Could you check a few things on this model? Use its own coordinates, in mm. A direction names the side the tool comes from. Give positions to 0.01 mm unless a question says otherwise; leave off trailing zeros. Loops run counter-clockwise (first coordinate to the right, second up) from the corner with the lowest first, then second, coordinate; pieces in that order, holes last. Notation, with made-up numbers: M -16,60.5 L 14,60.5 A20 ccw 14,91.5 Z; hole C 15,-40 d10. An arc over 180 degrees is marked long. Answer in a Markdown table with one row per item. Add a question column.
1. Which directions (+Z, -Z, +X, -X, +Y, -Y) give clear straight access to the entire face, cutting with the end or side of a thin tool? Please do faces 4 (the flat face through (0, -9.994, -12)), 5 (the flat face through (-2, -6.494, 23)), 6 (the flat face through (24, -9, -3.544)).
2. I need wall thicknesses on line 1 along X through (y, z) = (-8.25, 17.5); line 2 along Z through (x, y) = (15.25, -7.05); line 3 along Z through (x, y) = (-18.5, -7.05). Which ranges of each line are inside material? Lowest first, please. Write a range as from..to.
3. If we section it at D-D on x = -19: List the corners of the cut face in (y, z) for me, then the cut area to 3 significant figures.
4. If we section it at B-B on z = 0: List the corners of the cut face in (x, y) for me (3 decimals).
5. If we section it at C-C on y = -9: List the corners of the cut face in (x, z) for me (3 decimals).
6. I'm going to push flat-ended pins straight in: pin 1 Ø2.5 at (x, y) = (-24.5, -10) entering from -Z; pin 2 Ø3.5 at (x, y) = (23.5, -9.5) entering from -Z; pin 3 Ø1.5 at (x, y) = (23.5, -10) entering from +Z. Where does each tip first touch, or does it pass through?
7. Thinking about a two-plate mould opening in X: for faces 1 (the flat face through (24, -10, 3.456)), 2 (the flat face through (10, -11.5, -19)), 3 (the cylindrical face through (-24.68, -13.34, -7.77)), which applies, released by +X, released by -X, zero draft, split by the parting line, or undercut?
8. If we section it at A-A on x = 0: List the corners of the cut face in (y, z) for me (3 decimals), then the cut area to 3 significant figures.
Autodesk Inventor part; units mm, degrees
ref_plane "Work Plane1" through (-28, 0, 0) normal (1, 0, 0) x (0, 1, 0)
ref_plane "Work Plane2" through (28, 0, 0) normal (1, 0, 0) x (0, 1, 0)
ref_plane "XZ Plane" through (0, 0, 0) normal (0, 1, 0) x (-1, 0, 0)
sketch "Sketch2" plane through (0, 0, 0) normal (0, 0, 1) x (1, 0, 0)
  line L0 (0, 0) -> (-20.875, 0)
  line L1 (-20.875, 0) -> (-20.875, -11.5)
  line L2 (-20.875, -11.5) -> (-22.875, -11.5)
  line L3 (-22.875, -11.5) -> (-22.875, -6.4943)
  line L4 (-22.875, -6.4943) -> (-25.875, -6.4943)
  line L5 (-25.875, -6.4943) -> (-25.875, -12.9943)
  line L6 (0, -3) -> (0, 0)
  line L7 (-25.875, -12.9943) -> (-25.875, -19.9943)
  line L8 (-25.875, -19.9943) -> (-14.1, -19.9943)
  line L9 (-14.1, 0) -> (-14.1, -19.9943) construction
  line L10 (-7.6, 0) -> (-7.6, -3) construction
  line L11 (-7.6, -3) -> (0, -3) construction
  line L12 (-7.6, 0) -> (-7.6, -10) construction
  line L13 (-8.349, -3) -> (-14.1, -3)
  line L14 (-14.1, -19.9943) -> (-14.1, -3)
  line L15 (-11.6, -3) -> (-11.6, -9.9943)
  line L16 (-11.6, -9.9943) -> (-14.1, -9.9943)
  line L17 (-7.6, 0) -> (-8.349, -3)
  dimension "d3" = 20.875
  dimension "d4" = 11.5
  dimension "d5" = 2
  dimension "d6" = 3
  dimension "d7" = 6.5
  dimension "d9" = 7
  dimension "d10" = 14.1
  dimension "d11" = 3
  dimension "d12" = 7.6
  dimension "d13" = 10
  dimension "d31" = 2.5
  dimension "d33" = 10
revolve "Revolution1" add sketch "Sketch2" angle 360 about axis through (0, -3, 0) along (0, 1, 0)
sketch "Sketch3" plane through (0, 0, 0) normal (1, 0, 0) x (0, 1, 0)
  line L0 (0, -7.6) -> (0, 7.6)
  circle A0 centre (-7.05, 0) radius 3.5
  point P0 (0, 0)
  dimension "d16" = 7.05
  dimension "d17" = 0
  dimension "d20" = 7
extrude "Extrusion1" cut sketch "Sketch3" along normal through all both and the other way through all
ref_plane "Work Plane1" through (-28, 0, 0) normal (1, 0, 0) x (0, 1, 0)
sketch "Sketch4" plane through (-28, 0, 0) normal (1, 0, 0) x (0, 1, 0)
  line L0 (-11.5, -20.875) -> (-11.5, 20.875)
  line L1 (-6.4943, -3.4556) -> (-11.5, -3.4556)
  line L2 (-11.5, -3.4556) -> (-11.5, 3.5444)
  line L3 (-11.5, 3.5444) -> (-6.4943, 3.5444)
  line L4 (-6.4943, 3.5444) -> (-6.4943, -3.4556)
  point P0 (0, 0)
  dimension "d24" = 7
extrude "Extrusion2" cut sketch "Sketch4" along normal up to surface
ref_plane "Work Plane2" through (28, 0, 0) normal (1, 0, 0) x (0, 1, 0)
sketch "Sketch5" plane through (28, 0, 0) normal (1, 0, 0) x (0, 1, 0)
  line L0 (-11.5, -20.875) -> (-11.5, 20.875)
  line L1 (-6.4943, 3.4556) -> (-11.5, 3.4556)
  line L2 (-11.5, 3.4556) -> (-11.5, -3.5444)
  line L3 (-11.5, -3.5444) -> (-6.4943, -3.5444)
  line L4 (-6.4943, -3.5444) -> (-6.4943, 3.4556)
  point P0 (0, 0)
  dimension "d28" = 7
extrude "Extrusion3" cut sketch "Sketch5" against normal up to surface
properties part number "bottom seal v2"
Results:
| question | item | result |
|---|---|---|
| 1 | face 4 | -Y |
| 1 | face 5 | +Z, +Y |
| 1 | face 6 | +X, +Y |
| 2 | line 1 | -19.06..-14.73, -11.38..11.38, 14.73..19.06 |
| 2 | line 2 | -20.9..-17.05, -14.25..-3.5, 3.5..14.25, 17.05..20.9 |
| 2 | line 3 | -18.09..-13.45, -9.67..-3.5, 3.5..9.67, 13.45..18.09 |
| 3 | outline | M -19.99,-17.56 L -6.49,-17.56 L -6.49,-12.74 L -11.5,-12.74 L -11.5,-8.65 L 0,-8.65 L 0,8.65 L -11.5,8.65 L -11.5,12.74 L -6.49,12.74 L -6.49,17.56 L -19.99,17.56 Z; hole C -7.05,0 d7 |
| 3 | area | 507 mm2 |
| 4 | outline | M -25.875,-19.994 L -14.1,-19.994 L -14.1,-10.55 L -20.875,-10.55 L -20.875,-11.5 L -25.875,-11.5 Z; M -20.875,-3.55 L -11.6,-3.55 L -11.6,-3 L -8.349,-3 L -7.6,0 L -20.875,0 Z; M 7.6,0 L 8.349,-3 L 11.6,-3 L 11.6,-3.55 L 20.875,-3.55 L 20.875,0 Z; M 14.1,-19.994 L 25.875,-19.994 L 25.875,-11.5 L 20.875,-11.5 L 20.875,-10.55 L 14.1,-10.55 Z |
| 5 | outline | M -25.643,-3.456 A25.875 ccw 25.631,-3.544 L 22.599,-3.544 A22.875 cw -22.612,-3.456 Z; M -25.631,3.544 L -22.599,3.544 A22.875 cw 22.612,3.456 L 25.643,3.456 A25.875 ccw Z; M -20.672,-2.906 A20.875 ccw 20.672,-2.906 L 11.23,-2.906 A11.6 cw -11.23,-2.906 Z; M -20.672,2.906 L -11.23,2.906 A11.6 cw 11.23,2.906 L 20.672,2.906 A20.875 ccw Z |
| 6 | pin 1 | z = -11.36 |
| 6 | pin 2 | z = -14.02 |
| 6 | pin 3 | z = 12.33 |
| 7 | face 1 | zero draft |
| 7 | face 2 | undercut |
| 7 | face 3 | split by the parting line |
| 8 | outline | M -19.994,-25.875 L -6.494,-25.875 L -6.494,-22.875 L -11.5,-22.875 L -11.5,-20.875 L 0,-20.875 L 0,-7.6 L -3,-8.349 L -3,-11.6 L -9.994,-11.6 L -9.994,-14.1 L -19.994,-14.1 Z; M -19.994,14.1 L -9.994,14.1 L -9.994,11.6 L -3,11.6 L -3,8.349 L 0,7.6 L 0,20.875 L -11.5,20.875 L -11.5,22.875 L -6.494,22.875 L -6.494,25.875 L -19.994,25.875 Z |
| 8 | area | 458 mm2 |
